Build history of the part. All positions in model axes, mm. Give positions to 0.01 mm unless a question says otherwise; leave off trailing zeros. Write each loop counter-clockwise with the first axis right and the second up, starting at its lowest first coordinate (ties: lowest second). Pieces come first, ordered by that corner, then holes. Notation, with made-up numbers: (-9, 35.25) -> (20, 35.25) arc R25 cw to (20, 73.25) -> close; hole circle Ø9 at (55, 34). An arc over 180 degrees is marked (long way). One line per question, with ' | ' between items. Start each with the question number.
(1) Band-saw the part on C-C, the plane y = 4.25. Count the separate pieces of the cut face and the enclosed holes in it, and give its area (3 significant figures).
(2) Pin check, flat tip, straight feed: P1, Ø9, axis at x = 485, z = 82.5, coming from the -Y side. Stop position of the tip, or through.
(3) Band-saw the part on B-B, the plane x = 435.5. Give the cut face in (y, z).
(4) Band-saw the part on A-A, the plane z = 22. Give the cut face in (x, y), and give its area (3 significant figures).
(5) Drill centre lines: probe 1 along X at (y, z) = (2, 0); probe 2 along Z at (x, y) = (175, 4); probe 3 along X at (y, z) = (5, -82.5). Where is each one in solid material? Low to high. Write a range as from..to.
(6) Pull direction X, two halves, no side cores. Call faces 1 (the flat face through (229, 0, -2)), 2 (the cylindrical face through (549.447, 3.944, -8.462)): released by +X, released by -X, zero draft, split by the parting line, or undercut.
from build123d import *

# Parameters (mm, degrees)
SKETCH1_W           = 820
SKETCH1_H           = 320
SKETCH1_R           = 75
SKETCH1_R_2         = 5.5
SKETCH1_R_3         = 65
BOSS_EXTRUDE1_DEPTH = 8
SKETCH2_R           = 5.5
CUT_EXTRUDE2_DEPTH  = 10


with BuildPart() as part:
    # Sketch1 → Boss-Extrude1 (new body)
    with BuildSketch(Plane(origin=(0, 0, 0), x_dir=(1, 0, 0), z_dir=(0, 1, 0))):
        with Locations((235, 0)):
            Rectangle(SKETCH1_W, SKETCH1_H)
        with Locations(Location((0, 0, 0), (0, 0, 270))):
            Circle(SKETCH1_R, mode=Mode.SUBTRACT)
        with Locations(Location((0, -98, 0), (0, 0, 270))):
            Circle(SKETCH1_R_2, mode=Mode.SUBTRACT)
        with Locations(Location((-84.870489571, -49, 0), (0, 0, 270))):
            Circle(SKETCH1_R_2, mode=Mode.SUBTRACT)
        with Locations(Location((-84.870489571, 49, 0), (0, 0, 270))):
            Circle(SKETCH1_R_2, mode=Mode.SUBTRACT)
        with Locations(Location((0, 98, 0), (0, 0, 270))):
            Circle(SKETCH1_R_2, mode=Mode.SUBTRACT)
        with Locations(Location((84.870489571, 49, 0), (0, 0, 270))):
            Circle(SKETCH1_R_2, mode=Mode.SUBTRACT)
        with Locations(Location((84.870489571, -49, 0), (0, 0, 270))):
            Circle(SKETCH1_R_2, mode=Mode.SUBTRACT)
        with Locations(Location((485, 0, 0), (0, 0, 270))):
            Circle(SKETCH1_R_3, mode=Mode.SUBTRACT)
        with Locations(Location((567.5, 0, 0), (0, 0, 270))):
            Circle(SKETCH1_R_2, mode=Mode.SUBTRACT)
        with Locations(Location((485, -82.5, 0), (0, 0, 270))):
            Circle(SKETCH1_R_2, mode=Mode.SUBTRACT)
        with Locations(Location((402.5, 0, 0), (0, 0, 270))):
            Circle(SKETCH1_R_2, mode=Mode.SUBTRACT)
        with Locations(Location((485, 82.5, 0), (0, 0, 270))):
            Circle(SKETCH1_R_2, mode=Mode.SUBTRACT)
    extrude(amount=BOSS_EXTRUDE1_DEPTH)

    # Sketch2 → Cut-Extrude2 (cut)
    with BuildSketch(Plane(origin=(0, 0, 0), x_dir=(1, 0, 0), z_dir=(0, 1, 0))):
        with Locations(Location((175, -60, 0), (0, 0, 270))):
            Circle(SKETCH2_R)
        with Locations(Location((175, -100, 0), (0, 0, 270))):
            Circle(SKETCH2_R)
        with Locations(Location((368, -100, 0), (0, 0, 270))):
            Circle(SKETCH2_R)
        with Locations(Location((368, -60, 0), (0, 0, 270))):
            Circle(SKETCH2_R)
    extrude(amount=CUT_EXTRUDE2_DEPTH, mode=Mode.SUBTRACT)


solid = part.part
Results:
1) separate pieces: 1 | enclosed holes: 16 | area: 230,000 mm²
2) P1: passes through
3) outline: (0, -160) -> (8, -160) -> (8, -42.13) -> (0, -42.13) -> close; (0, 42.13) -> (8, 42.13) -> (8, 160) -> (0, 160) -> close
4) outline: (-175, 0) -> (-71.7, 0) -> (-71.7, 8) -> (-175, 8) -> close; (71.7, 0) -> (423.84, 0) -> (423.84, 8) -> (71.7, 8) -> close; (546.16, 0) -> (645, 0) -> (645, 8) -> (546.16, 8) -> close | area: 4,430 mm²
5) probe 1: x = -175..-75, 75..397, 408..420, 550..562, 573..645 | probe 2: z = -160..54.5, 65.5..94.5, 105.5..160 | probe 3: x = -175..479.5, 490.5..645
6) face 1: zero draft | face 2: undercut
